Part model, mm, in its own coordinate system. Face numbers are marked on the shaded views. A direction names the side the tool comes from. Coordinates: 2 decimals unless noted, no trailing zeros. Order: outer loops, then holes, each group sorted by start corner. A loop starts at its lowest first (then second) coordinate and runs counter-clockwise, first axis right, second up.
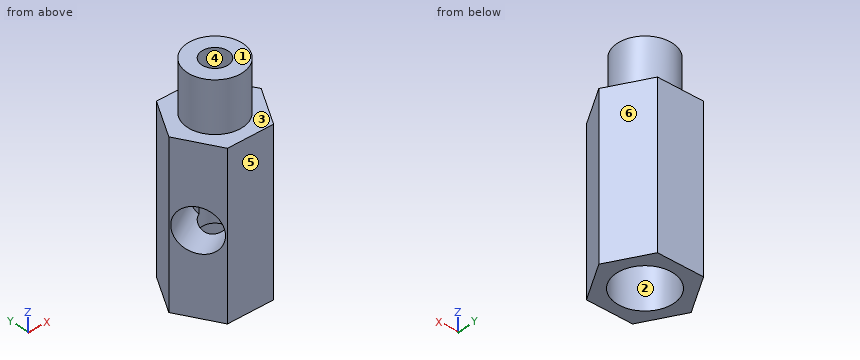
```python
from build123d import *

# Parameters (mm, degrees)
BOSS_EXTRUDE1_DEPTH = 50.8
SKETCH4_R           = 3.175
CUT_EXTRUDE2_DEPTH  = 51.8
SKETCH2_R           = 6.635
CUT_EXTRUDE1_DEPTH  = 12.065
SKETCH3_R           = 6.86
CUT_EXTRUDE3_DEPTH  = 12.065
SKETCH5_R           = 5.145
CUT_EXTRUDE4_DEPTH  = 10


with BuildPart() as part:
    # Sketch1 → Boss-Extrude1 (new body)
    with BuildSketch(Plane(origin=(0, 0, 0), x_dir=(0, 1, 0), z_dir=(0, 0, 1))):
        Polygon((9.525, -5.499261314), (9.525, 5.499261314), (0, 10.998522628), (-9.525, 5.499261314), (-9.525, -5.499261314), (0, -10.998522628), align=None)
    extrude(amount=BOSS_EXTRUDE1_DEPTH)

    # Sketch4 → Cut-Extrude2 (cut, through all)
    with BuildSketch(Plane.XY.offset(50.8)):
        Circle(SKETCH4_R)
    extrude(amount=-CUT_EXTRUDE2_DEPTH, mode=Mode.SUBTRACT)

    # Sketch2 → Cut-Extrude1 (cut)
    with BuildSketch(Plane.XY.offset(50.8)):
        Polygon((10.998522628, 0), (5.499261314, 9.525), (-5.499261314, 9.525), (-10.998522628, 0), (-5.499261314, -9.525), (5.499261314, -9.525), align=None)
        Circle(SKETCH2_R, mode=Mode.SUBTRACT)
    extrude(amount=-CUT_EXTRUDE1_DEPTH, mode=Mode.SUBTRACT)

    # Sketch3 → Cut-Extrude3 (cut)
    with BuildSketch(Plane(origin=(0, 0, 0), x_dir=(1, 0, 0), z_dir=(0, 0, -1))):
        Circle(SKETCH3_R)
    extrude(amount=-CUT_EXTRUDE3_DEPTH, mode=Mode.SUBTRACT)

    # Sketch5 → Cut-Extrude4 (cut)
    with BuildSketch(Plane(origin=(-8.248891971, -4.7625, 0), x_dir=(0.5, -0.866025404, 0), z_dir=(-0.866025404, -0.5, 0))):
        with Locations((0, 19.3675)):
            Circle(SKETCH5_R)
    extrude(amount=-CUT_EXTRUDE4_DEPTH, mode=Mode.SUBTRACT)


solid = part.part
```
(1) Probe line 1 (X direction, y = 0, z = 8); line 2 (Y direction, x = 0, z = 3.25) (3 decimals); line 3 (Z direction, x = 3.25, y = -2.5) (3 decimals). List the from-to ranges inside material, lowest first.
(2) Slice it at A-A, the plane z = 25.5. Give the cut face in (x, y) (3 decimals).
(3) Slice it at B-B, the plane z = 7.5. Give the cut face in (x, y) (3 decimals).
(4) Drop flat-ended pins along their axis: pin 1 (3 mm diameter, centred on y = -1, z = 32.5, fed in from -X); pin 2 (5 mm diameter, centred on y = -5, z = 27, fed in from +X); pin 3 (4 mm diameter, centred on x = 1.5, y = -2, fed in from -Z) (3 decimals); pin 4 (4 mm diameter, centred on x = 0, y = 0, fed in from -Z). Give the stop position or say it passes through.
(5) Slice it at C-C, the plane y = -0.5. State how many separate pieces and enclosed holes the cut face has, then the cut area to 3 significant figures.
(6) Slice it at D-D, the plane z = 18.5. Give the cut face in (x, y) (3 decimals), then the cut area to 3 significant figures.
(7) Tool access for the marked faces 1, 2 and 3: list every direction of +Z, -Z, +X, -X, +Y, -Y with a clear straight run to the whole face (end or side of a thin tool).
(8) Pull direction X, two halves, no side cores. Call the marked faces 4, 5 and 6: +X half, -X half, draft (parallel to the pull), parting line (faces both ways), or undercut.
Here are the results:
1. line 1: x = -11 to -6.86, 6.86 to 11
1. line 2: y = -9.525 to -6.86, 6.86 to 9.525
1. line 3: z = 12.065 to 50.8
2. outline: (-10.999, 0) - (-5.499, -9.525) - (5.499, -9.525) - (10.999, 0) - (5.499, 9.525) - (-5.499, 9.525) - close; hole circle Ø6.35 at (0, 0)
3. outline: (-10.999, 0) - (-5.499, -9.525) - (5.499, -9.525) - (10.999, 0) - (5.499, 9.525) - (-5.499, 9.525) - close; hole circle Ø13.72 at (0, 0)
4. pin 1: stops at x = -11
4. pin 2: stops at x = 9.56
4. pin 3: stops at z = 12.065
4. pin 4: passes through
5. separate pieces: 3
5. enclosed holes: 0
5. area: 522 mm2
6. outline: (-10.999, 0) - (-10.785, -0.371) - (-2.124, 4.629) - (-1.158, 2.956) arc R3.175 cw to (1.981, -2.481) - (2.947, -4.154) - (-5.713, -9.154) - (-5.499, -9.525) - (5.499, -9.525) - (10.999, 0) - (5.499, 9.525) - (-5.499, 9.525) - close
6. area: 200 mm2
7. face 1: +Z, +X, -X, +Y, -Y
7. face 2: -Z
7. face 3: +Z
8. face 4: undercut
8. face 5: draft
8. face 6: +X half
